from build123d import *

# Parameters (mm, degrees)
SKETCH15_R               = 11
BOSS_EXTRUDE4_DEPTH      = 50.8
CUT_EXTRUDE9_DEPTH       = 25.4
CUT_EXTRUDE9_DEPTH_BACK  = 50.8
SKETCH16_R               = 5
SKETCH17_R               = 2.5
CUT_EXTRUDE10_DEPTH      = 25.4
SKETCH20_W               = 0.929150013
SKETCH20_H               = 0.563484587
CUT_EXTRUDE11_DEPTH      = 25.4
SKETCH22_R               = 3.175
CUT_EXTRUDE14_DEPTH      = 12
CUT_EXTRUDE15_DEPTH      = 12.7
CUT_EXTRUDE15_DEPTH_BACK = 10
SKETCH33_R               = 11


with BuildPart() as part:
    # Sketch15 → Boss-Extrude4 (new body)
    with BuildSketch(Plane.XY):
        Circle(SKETCH15_R)
    extrude(amount=BOSS_EXTRUDE4_DEPTH)

    # Sketch16 → Cut-Extrude9 (cut, two sides: drawn at the far end of the back side and taken through both)
    with BuildSketch(Plane.XY.offset(-CUT_EXTRUDE9_DEPTH_BACK)):
        Circle(SKETCH16_R)
    extrude(amount=CUT_EXTRUDE9_DEPTH + CUT_EXTRUDE9_DEPTH_BACK, mode=Mode.SUBTRACT)

    # Sketch17 → Cut-Extrude10 (cut)
    with BuildSketch(Plane.XY.offset(50.8)):
        Circle(SKETCH17_R)
    extrude(amount=-CUT_EXTRUDE10_DEPTH, mode=Mode.SUBTRACT)

    # Sketch20 → Cut-Extrude11 (cut)
    with BuildSketch(Plane.XY.offset(50.8)):
        with Locations((-0.035424993, 2.498467219)):
            Rectangle(SKETCH20_W, SKETCH20_H)
    extrude(amount=-CUT_EXTRUDE11_DEPTH, mode=Mode.SUBTRACT)

    # Sketch22 → Cut-Extrude14 (cut)
    with BuildSketch(Plane(origin=(0, 0, 0), x_dir=(1, 0, 0), z_dir=(0, 1, 0))):
        with Locations(Location((0, -39.506560459, 0), (0, 0, 270))):
            Circle(SKETCH22_R)
    extrude(amount=-CUT_EXTRUDE14_DEPTH, mode=Mode.SUBTRACT)

    # Sketch33 → Cut-Extrude15 (cut, two sides: drawn at the far end of the back side and taken through both)
    with BuildSketch(Plane.XY.offset(-CUT_EXTRUDE15_DEPTH_BACK)):
        Circle(SKETCH33_R)
    extrude(amount=CUT_EXTRUDE15_DEPTH + CUT_EXTRUDE15_DEPTH_BACK, mode=Mode.SUBTRACT)


solid = part.part
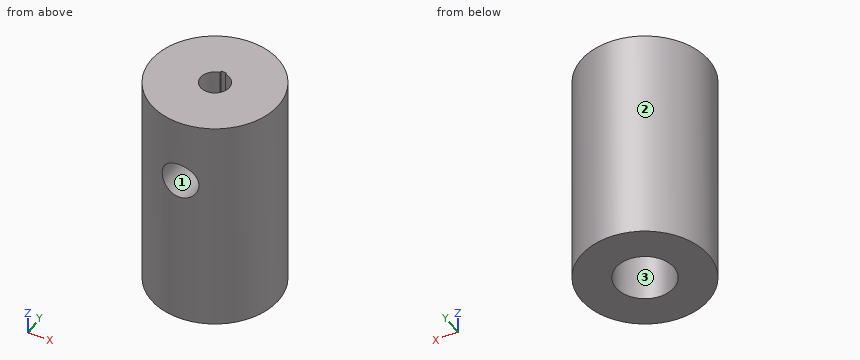
The listing builds one solid part. Answer for the finished solid, in the listing's coordinates (mm). Face numbers are marked on the shaded views. Give positions to 0.01 mm unless a question says otherwise; leave off trailing zeros. Write each loop counter-clockwise with the first axis right and the second up, starting at its lowest first coordinate (ties: lowest second). Pieces come first, ordered by that corner, then holes. Notation, with made-up numbers: (60.25, 7.5) - (107.25, 7.5) arc R18 ccw to (107.25, 42.5) - close; hole circle Ø9 at (35.5, 41). An arc over 180 degrees is marked (long way). One line per question, with ' | ' between items. Start each with the question number.
1. Straight lines are drawn through the part: line 1 (Y direction, x = 0, z = 31.25); line 2 (Z direction, x = 0, y = -7.25); line 3 (Z direction, x = 2, y = 3.5). For each, find the intervals that lie inside material, in ascending order.
2. Section B-B, the plane y = -2 is taken. Determine the outline of the cut face in (x, z) (3 decimals).
3. Given P1, Ø0.7, axis at x = 3, z = 40.5, coming from the -Y side; P2, Ø12, axis at x = -5, z = 39.5, coming from the -Y side; P3, Ø2, axis at x = 2.5, z = 33, coming from the -Y side; P4, Ø1, axis at y = -2.5, z = 45.5, coming from the +X side, each flat-ended and moving along its own axis, determine where each tip first touches the part or whether it passes through.
4. Section D-D, the plane y = -4.25 is taken. Determine the outline of the cut face in (x, z) (3 decimals).
5. Section C-C, the plane z = 45 is taken. Determine the outline of the cut face in (x, y), then the cut area to 3 significant figures.
6. Section A-A, the plane x = 0 is taken. Determine the outline of the cut face in (y, z).
7. Determine the mould class of the marked faces 1, 2 and 3 for opening direction Y: +Y half, -Y half, draft (parallel to the pull), parting line (faces both ways), or undercut.
Result:
1) line 1: y = -11 to -2.5, 2.78 to 11 | line 2: z = 12.7 to 36.33, 42.68 to 50.8 | line 3: z = 25.4 to 50.8
2) outline: (-10.817, 12.7) - (-4.583, 12.7) - (-4.583, 25.4) - (-1.5, 25.4) - (-1.5, 36.708) arc R3.175 cw to (-1.5, 42.305) - (-1.5, 50.8) - (-10.817, 50.8) - close; (1.5, 25.4) - (4.583, 25.4) - (4.583, 12.7) - (10.817, 12.7) - (10.817, 50.8) - (1.5, 50.8) - (1.5, 42.305) arc R3.175 cw to (1.5, 36.708) - close
3) P1: stops at y = -10.61 | P2: stops at y = -11 | P3: stops at y = -10.9 | P4: stops at x = 10.82
4) outline: (-10.146, 12.7) - (-2.634, 12.7) - (-2.634, 25.4) - (2.634, 25.4) - (2.634, 12.7) - (10.146, 12.7) - (10.146, 50.8) - (-10.146, 50.8) - close; hole circle Ø6.35 at (0, 39.507)
5) outline: circle Ø22 at (0, 0); hole (-0.5, 2.45) arc R2.5 ccw (long way) to (0.43, 2.46) - (0.43, 2.78) - (-0.5, 2.78) - close | area: 360 mm2
6) outline: (-11, 12.7) - (-5, 12.7) - (-5, 25.4) - (-2.5, 25.4) - (-2.5, 36.33) - (-11, 36.33) - close; (-11, 42.68) - (-2.5, 42.68) - (-2.5, 50.8) - (-11, 50.8) - close; (2.78, 25.4) - (5, 25.4) - (5, 12.7) - (11, 12.7) - (11, 50.8) - (2.78, 50.8) - close
7) face 1: draft | face 2: parting line | face 3: undercut
